Autodesk Inventor part; units mm, degrees
ref_plane "YZ Plane" through (0, 0, 0) normal (1, 0, 0) x (0, 1, 0)
ref_plane "XZ Plane" through (0, 0, 0) normal (0, 1, 0) x (-1, 0, 0)
ref_plane "XY Plane" through (0, 0, 0) normal (0, 0, 1) x (1, 0, 0)
sketch "Sketch1" plane through (0, 0, 0) normal (0, 0, 1) x (1, 0, 0)
  line L0 (-63.5, -190.5) -> (63.5, -190.5)
  line L1 (63.5, -190.5) -> (63.5, 190.5) construction
  line L2 (63.5, 190.5) -> (-63.5, 190.5) construction
  line L3 (-63.5, 190.5) -> (-63.5, -190.5)
  line L4 (-63.5, -190.5) -> (63.5, 190.5) construction
  line L5 (63.5, -190.5) -> (-63.5, 190.5) construction
  line L6 (-63.5, 190.5) -> (-6.35, 0)
  line L7 (-6.35, 0) -> (63.5, -190.5)
  line L8 (-63.5, -190.5) -> (-66.675, -190.5)
  line L9 (-66.675, -190.5) -> (-66.675, -12.7)
  line L10 (-66.675, -12.7) -> (-63.5, -12.7)
  line L11 (-63.5, -12.7) -> (-63.5, -190.5)
  line L12 (-63.5, 0) -> (-66.675, 0)
  line L13 (-66.675, 0) -> (-66.675, 177.8)
  line L14 (-66.675, 177.8) -> (-63.5, 177.8)
  line L15 (-63.5, 177.8) -> (-63.5, 0)
  point P0 (0, 0)
  dimension "d0" = 381
  dimension "d1" = 127
  dimension "d2" = 190.5
  dimension "d3" = 57.15
  dimension "d7" = 3.175
  dimension "d8" = 177.8
  dimension "d9" = 3.175
  dimension "d10" = 12.7
  dimension "d11" = 12.7
extrude "Extrusion1" add sketch "Sketch1" along normal blind 9.525
equation "\"d2\" = 0.5 * d0"
properties part number "Fin"
Verification items for the finished model (mm, model axes). A direction names the side the tool comes from. Coordinates: 2 decimals unless noted, no trailing zeros. Loops run counter-clockwise (first coordinate to the right, second up) from the corner with the lowest first, then second, coordinate; pieces in that order, holes last. Notation, with made-up numbers: (9, 66) -> (38, 66) arc R21 cw to (38, 105) -> close; hole circle Ø1 at (-36, 87). An arc over 180 degrees is marked (long way). Answer as a JSON object with one key per item and string values. Group by question number.
Item 1: Depth check by flat-ended pin: pin 1 (4 mm diameter, centred on y = -41, z = 4.5, fed in from +X); pin 2 (3 mm diameter, centred on y = -5.5, z = 4.5, fed in from -X). Enter the tip coordinate at first touch or a pass-through.
Item 2: Tool access check on faces 1 (the flat face through (-2, -190.5, 5)), 2 (the flat face through (-63.5, 184, 5)). Record the directions out of +Z, -Z, +X, -X, +Y, -Y that give a thin tool (end or side, any length) a straight path to the whole face; none if there is none.
Item 3: Mould release check, pull along Y, two halves, no side actions. Record for faces 3 (the flat face through (28.086, -93.917, 4.696)), 4 (the flat face through (-66.675, -103, 5)), 5 (the flat face through (-63.5, -6, 5)): +Y half, -Y half, draft (parallel to the pull), parting line (faces both ways), or undercut.
Item 4: Sectioned sample at A-A on z = 6.75. Record the boundary of the cut face in (x, y) (3 decimals).
Item 5: Scan lines: probe 1 along X at (y, z) = (-153, 2) (3 decimals); probe 2 along X at (y, z) = (24, 5.5) (3 decimals). Record each from-to range of solid material in increasing order.
Item 6: Sectioned sample at B-B on y = 41. Record the boundary of the cut face in (x, z) (3 decimals), plus the area to 3 significant figures.
Item 7: Sectioned sample at C-C on x = 47. Record the boundary of the cut face in (y, z) (3 decimals).
Evaluation:
{
 "1": {"pin 1": "stops at x = 9.42", "pin 2": "stops at x = -63.5"},
 "2": {"face 1": "+Z, -Z, +X, -X, -Y", "face 2": "+Z, -Z, -X, +Y"},
 "3": {"face 3": "+Y half", "face 4": "draft", "face 5": "undercut"},
 "4": {"outline": "(-66.675, -190.5) -> (63.5, -190.5) -> (-6.35, 0) -> (-63.5, 190.5) -> (-63.5, 177.8) -> (-66.675, 177.8) -> (-66.675, 0) -> (-63.5, 0) -> (-63.5, -12.7) -> (-66.675, -12.7) -> close"},
 "5": {"probe 1": "x = -66.675 to 49.75", "probe 2": "x = -66.675 to -13.55"},
 "6": {"outline": "(-66.675, 0) -> (-18.65, 0) -> (-18.65, 9.525) -> (-66.675, 9.525) -> close", "area": "457 mm²"},
 "7": {"outline": "(-190.5, 0) -> (-145.5, 0) -> (-145.5, 9.525) -> (-190.5, 9.525) -> close"}
}
